Geometry check sheet. Reference: the model listing, model coordinates, mm. A direction names the side the tool comes from. Give positions to 0.01 mm unless a question says otherwise; leave off trailing zeros. Loops run counter-clockwise (first coordinate to the right, second up) from the corner with the lowest first, then second, coordinate; pieces in that order, holes last.
```python
from build123d import *

# Parameters (mm, degrees)
BOSS_EXTRU_1_DEPTH                                = 30
ESQUISSE6_W                                       = 37
ESQUISSE6_H                                       = 37.5
BOSS_EXTRU_4_DEPTH                                = 18
ESQUISSE7_R                                       = 6.375
BOSS_EXTRU_5_DEPTH                                = 10
ESQUISSE8_R                                       = 1.5
ENL_V_MAT_EXTRU_1_DEPTH                           = 43
ESQUISSE9_W                                       = 10
ESQUISSE9_H                                       = 10
ENL_V_MAT_EXTRU_2_DEPTH                           = 10
ESQUISSE10_W                                      = 10
ESQUISSE10_H                                      = 7
ENL_V_MAT_EXTRU_5_DEPTH                           = 10
ESQUISSE11_W                                      = 10
ESQUISSE11_H                                      = 7
ENL_V_MAT_EXTRU_6_DEPTH                           = 10
ESQUISSE12_W                                      = 20
ESQUISSE12_H                                      = 37.154688963
ENL_V_MAT_EXTRU_7_DEPTH                           = 19.44
ESQUISSE13_W                                      = 10
ESQUISSE13_H                                      = 10
ENL_V_MAT_EXTRU_8_DEPTH                           = 9.801191536
ESQUISSE14_W                                      = 37
ESQUISSE14_H                                      = 17.5
BOSS_EXTRU_6_DEPTH                                = 5
ESQUISSE20_W                                      = 10
ESQUISSE20_H                                      = 5
BOSS_EXTRU_8_DEPTH                                = 10
FRAISAGE_POUR_VIS_T_TE_FRAIS_E_BOMB_E_D           = 3.4
FRAISAGE_POUR_VIS_T_TE_FRAIS_E_BOMB_E_DEPTH       = 5
FRAISAGE_POUR_VIS_T_TE_FRAIS_E_BOMB_E_CSINK_D     = 6.3
FRAISAGE_POUR_VIS_T_TE_FRAIS_E_BOMB_E_CSINK_ANGLE = 90
FRAISAGE_POUR_VIS_T_TE_FRAIS_E_BOMB_E_TIP         = 1.021463052


with BuildPart() as part:
    # Esquisse3 → Boss.-Extru.1 (new body)
    with BuildSketch(Plane(origin=(0, 0, 0), x_dir=(1, 0, 0), z_dir=(0, 1, 0))):
        Polygon((0, 0), (0, 55), (38, 55), (38, 37.5), (75, 37.5), (75, 0), align=None)
    extrude(amount=BOSS_EXTRU_1_DEPTH)

    # Esquisse6 → Boss.-Extru.4 (add)
    with BuildSketch(Plane(origin=(0, 30, 0), x_dir=(1, 0, 0), z_dir=(0, 1, 0))):
        with Locations((56.5, 18.75)):
            Rectangle(ESQUISSE6_W, ESQUISSE6_H)
    extrude(amount=BOSS_EXTRU_4_DEPTH)

    # Esquisse7 → Boss.-Extru.5 (add)
    with BuildSketch(Plane(origin=(0, 48, 0), x_dir=(1, 0, 0), z_dir=(0, 1, 0))):
        with Locations(Location((56.5, 19, 0), (0, 0, 270))):
            Circle(ESQUISSE7_R)
    extrude(amount=BOSS_EXTRU_5_DEPTH)

    # Esquisse8 → Enlèv. mat.-Extru.1 (cut)
    with BuildSketch(Plane(origin=(0, 48, 0), x_dir=(1, 0, 0), z_dir=(0, 1, 0))):
        with Locations(Location((43, 32.5, 0), (0, 0, 270))):
            Circle(ESQUISSE8_R)
        with Locations(Location((70, 32.5, 0), (0, 0, 270))):
            Circle(ESQUISSE8_R)
        with Locations(Location((70, 5, 0), (0, 0, 270))):
            Circle(ESQUISSE8_R)
        with Locations(Location((43, 5, 0), (0, 0, 270))):
            Circle(ESQUISSE8_R)
    extrude(amount=-ENL_V_MAT_EXTRU_1_DEPTH, mode=Mode.SUBTRACT)

    # Esquisse9 → Enlèv. mat.-Extru.2 (cut)
    with BuildSketch(Plane(origin=(75, 0, 0), x_dir=(0, 0, -1), z_dir=(1, 0, 0))):
        with Locations((5, 18)):
            Rectangle(ESQUISSE9_W, ESQUISSE9_H)
        with Locations((32.5, 18)):
            Rectangle(ESQUISSE9_W, ESQUISSE9_H)
    extrude(amount=-ENL_V_MAT_EXTRU_2_DEPTH, mode=Mode.SUBTRACT)

    # Esquisse10 → Enlèv. mat.-Extru.5 (cut)
    with BuildSketch(Plane(origin=(0, 0, -37.5), x_dir=(-1, 0, 0), z_dir=(0, 0, -1))):
        with Locations((-43, 16.5)):
            Rectangle(ESQUISSE10_W, ESQUISSE10_H)
    extrude(amount=-ENL_V_MAT_EXTRU_5_DEPTH, mode=Mode.SUBTRACT)

    # Esquisse11 → Enlèv. mat.-Extru.6 (cut)
    with BuildSketch(Plane.XY):
        with Locations((43, 16.5)):
            Rectangle(ESQUISSE11_W, ESQUISSE11_H)
    extrude(amount=-ENL_V_MAT_EXTRU_6_DEPTH, mode=Mode.SUBTRACT)

    # Esquisse12 → Enlèv. mat.-Extru.7 (cut)
    with BuildSketch(Plane(origin=(0, 30, 0), x_dir=(1, 0, 0), z_dir=(0, 1, 0))):
        with Locations((20, 26.621463983)):
            Rectangle(ESQUISSE12_W, ESQUISSE12_H)
    extrude(amount=-ENL_V_MAT_EXTRU_7_DEPTH, mode=Mode.SUBTRACT)

    # Esquisse13 → Enlèv. mat.-Extru.8 (cut)
    with BuildSketch(Plane.XY.offset(-45.198808464)):
        with Locations((20, 15.56)):
            Rectangle(ESQUISSE13_W, ESQUISSE13_H)
    extrude(amount=-ENL_V_MAT_EXTRU_8_DEPTH, mode=Mode.SUBTRACT)

    # Esquisse14 → Boss.-Extru.6 (add)
    with BuildSketch(Plane.XZ):
        with Locations((56.5, -46.25)):
            Rectangle(ESQUISSE14_W, ESQUISSE14_H)
    extrude(amount=-BOSS_EXTRU_6_DEPTH)

    # Esquisse20 → Boss.-Extru.8 (add)
    with BuildSketch(Plane.XY):
        with Locations((5, 2.5)):
            Rectangle(ESQUISSE20_W, ESQUISSE20_H)
    extrude(amount=BOSS_EXTRU_8_DEPTH)

    # Fraisage pour vis à tête fraisée bombée M32
    with Locations(Plane(origin=(0, 5, 0), x_dir=(1, 0, 0), z_dir=(0, 1, 0))):
        with Locations((5, -5), (47, 46), (66, 46)):
            CounterSinkHole(FRAISAGE_POUR_VIS_T_TE_FRAIS_E_BOMB_E_D / 2, FRAISAGE_POUR_VIS_T_TE_FRAIS_E_BOMB_E_CSINK_D / 2, depth=FRAISAGE_POUR_VIS_T_TE_FRAIS_E_BOMB_E_DEPTH, counter_sink_angle=FRAISAGE_POUR_VIS_T_TE_FRAIS_E_BOMB_E_CSINK_ANGLE)
            with Locations((0, 0, -(FRAISAGE_POUR_VIS_T_TE_FRAIS_E_BOMB_E_DEPTH + FRAISAGE_POUR_VIS_T_TE_FRAIS_E_BOMB_E_TIP / 2))):  # 118° drill point
                Cone(0, FRAISAGE_POUR_VIS_T_TE_FRAIS_E_BOMB_E_D / 2, FRAISAGE_POUR_VIS_T_TE_FRAIS_E_BOMB_E_TIP, mode=Mode.SUBTRACT)


solid = part.part
```
1) Sectioned sample at A-A on x = 66. Enter the section's corners in (y, z).
2) Sectioned sample at B-B on z = 5. Enter the section's corners in (x, y).
3) Scan lines: line 1 along Z through (x, y) = (70, 42); line 2 along X through (y, z) = (11.75, -32.5); line 3 along Y through (x, z) = (67.5, -30). Record each from-to range of solid material in increasing order.
4) Tool access check on faces 5 (the flat face through (30, 20, -26)), 6 (the flat face through (20, 20.56, -50)), 7 (the flat face through (56, 26, -37.5)). Record the directions out of +Z, -Z, +X, -X, +Y, -Y that give a thin tool (end or side, any length) a straight path to the whole face; none if there is none.
5) Sectioned sample at C-C on y = 34.5. Enter the section's corners in (x, z), plus the area to 3 significant figures.
6) Depth check by flat-ended pin: P1, Ø3, axis at x = 70, z = -33.5, coming from the +Y side; P2, Ø3, axis at x = 43, z = -6, coming from the -Y side; P3, Ø6, axis at x = 49, y = 11, coming from the -Z side; P4, Ø2.5, axis at x = 70, z = -32.5, coming from the +Y side. Enter the tip coordinate at first touch or a pass-through.
7) Mould release check, pull along X, two halves, no side actions. Record for faces 1 (the flat face through (43, 17, -27.5)), 2 (the flat face through (75, 24, -22)), 3 (the flat face through (71.2, 23, -3.8)), 4 (the flat face through (38, 39, -18)): +X half, -X half, draft (parallel to the pull), parting line (faces both ways), or undercut.
8) Sectioned sample at D-D on z = -9. Enter the section's corners in (x, y).
Determined:
1. outline: (0, -55) - (5, -55) - (5, -49.15) - (3.55, -47.7) - (0, -47.7) - close; (0, -44.3) - (3.55, -44.3) - (5, -42.85) - (5, -37.5) - (13, -37.5) - (13, -27.5) - (23, -27.5) - (23, -37.5) - (48, -37.5) - (48, 0) - (23, 0) - (23, -10) - (13, -10) - (13, 0) - (0, 0) - close
2. outline: (0, 0) - (3.3, 0) - (3.3, 3.55) - (1.85, 5) - (0, 5) - close; (6.7, 0) - (10, 0) - (10, 5) - (8.15, 5) - (6.7, 3.55) - close
3. line 1: z = -37.5 to -34, -31 to -6.5, -3.5 to 0
3. line 2: x = 0 to 10, 30 to 41.5, 44.5 to 68.5, 71.5 to 75
3. line 3: y = 0 to 13, 23 to 48
4. face 5: +Y
4. face 6: -Z
4. face 7: -Z, +X, +Y
5. outline: (38, -37.5) - (75, -37.5) - (75, 0) - (38, 0) - close; hole circle Ø3 at (43, -32.5); hole circle Ø3 at (43, -5); hole circle Ø3 at (70, -32.5); hole circle Ø3 at (70, -5)
5. area: 1,360 mm2
6. P1: stops at y = 48
6. P2: stops at y = 0
6. P3: stops at z = -37.5
6. P4: stops at y = 5
7. face 1: undercut
7. face 2: +X half
7. face 3: draft
7. face 4: -X half
8. outline: (0, 0) - (75, 0) - (75, 13) - (65, 13) - (65, 23) - (75, 23) - (75, 48) - (38, 48) - (38, 30) - (30, 30) - (30, 10.56) - (10, 10.56) - (10, 30) - (0, 30) - close; hole (38, 13) - (48, 13) - (48, 20) - (38, 20) - close
